```python
from build123d import *

# Parameters (mm, degrees)
BOSS_EXTRUDE1_DEPTH = 2.54
BOSS_EXTRUDE2_DEPTH = 2.54
SKETCH5_W           = 25.908
SKETCH5_H           = 34.036
BOSS_EXTRUDE3_DEPTH = 12.7
SKETCH6_R           = 1.27
BOSS_EXTRUDE4_DEPTH = 5.08
SKETCH7_W           = 5.08
SKETCH7_H           = 138.176
CUT_EXTRUDE1_DEPTH  = 2.54
CUT_EXTRUDE2_DEPTH  = 2.54


with BuildPart() as part:
    # Sketch1 → Boss-Extrude1 (new body)
    with BuildSketch(Plane(origin=(0, 0, 0), x_dir=(1, 0, 0), z_dir=(0, 1, 0))):
        Polygon((0, 0), (0, 152.4), (116.84, 152.4), (143.709327723, 0.01647018), align=None)
    extrude(amount=BOSS_EXTRUDE1_DEPTH)

    # Sketch2 → Boss-Extrude2 (add)
    with BuildSketch(Plane(origin=(0, 2.54, 0), x_dir=(1, 0, 0), z_dir=(0, 1, 0))):
        Polygon((117.220689951, 150.241), (2.159, 150.241), (2.159, 2.159), (143.331541909, 2.159), (142.435800847, 7.239), (7.239, 7.239), (7.239, 145.161), (118.116431013, 145.161), align=None)
    extrude(amount=BOSS_EXTRUDE2_DEPTH)

    # Sketch5 → Boss-Extrude3 (add)
    with BuildSketch(Plane.XZ):
        with Locations((44.90593, -61.477652)):
            Rectangle(SKETCH5_W, SKETCH5_H)
    extrude(amount=-BOSS_EXTRUDE3_DEPTH)

    # Sketch6 → Boss-Extrude4 (add)
    with BuildSketch(Plane(origin=(0, 12.7, 0), x_dir=(1, 0, 0), z_dir=(0, 1, 0))):
        with Locations((34.625191146, 75.319771658)):
            Circle(SKETCH6_R)
        with Locations((55.169983581, 75.290564093)):
            Circle(SKETCH6_R)
        with Locations((55.199191146, 49.284771658)):
            Circle(SKETCH6_R)
        with Locations((34.625191146, 49.284771658)):
            Circle(SKETCH6_R)
    extrude(amount=BOSS_EXTRUDE4_DEPTH)

    # Mirror2: part across plane


with BuildPart() as part_1:
    add(part.part)
    add(part.part.mirror(Plane(origin=(116.84, 2.54, -152.4), x_dir=(0.173648178, 0, 0.984807753), z_dir=(0.984807753, 0, -0.173648178))))

    # Sketch7 → Cut-Extrude1 (cut)
    with BuildSketch(Plane(origin=(0, 5.08, 0), x_dir=(1, 0, 0), z_dir=(0, 1, 0))):
        with Locations((4.699, 79.248)):
            Rectangle(SKETCH7_W, SKETCH7_H)
    extrude(amount=-CUT_EXTRUDE1_DEPTH, mode=Mode.SUBTRACT)

    # Sketch8 → Cut-Extrude2 (cut)
    with BuildSketch(Plane(origin=(0, 5.08, 0), x_dir=(1, 0, 0), z_dir=(0, 1, 0))):
        Polygon((86.740689951, 150.241), (86.740689951, 145.161), (118.116431013, 145.161), (140.439525591, 153.285941963), (138.702063263, 158.059580476), (117.220689951, 150.241), align=None)
    extrude(amount=-CUT_EXTRUDE2_DEPTH, mode=Mode.SUBTRACT)


solid = part_1.part
```
CAD build for the part. Positions are in the model's coordinates, mm. A direction names the side the tool comes from. Give positions to 0.01 mm unless a question says otherwise; leave off trailing zeros. Write each loop counter-clockwise with the first axis right and the second up, starting at its lowest first coordinate (ties: lowest second). Pieces come first, ordered by that corner, then holes. Notation, with made-up numbers: M 83,73.25 L 138,73.25 A12 cw 138,85.25 Z; hole C 78.5,31.5 d8. An arc over 180 degrees is marked long. Return JSON: item names as keys, results as strings. Group by question number.
(1) Band-saw the part on A-A (y = 8.5). Give the cut face in (x, z) (3 decimals), and give its area (3 significant figures).
(2) 3-axis set-ups, long thin cutter, end or side, ignore diameter. For faces 5 (the face through (210.59, 3.79, -26.64)), 6 (the face through (57.86, 8, -62)), 7 (the face through (250.312, 3.792, -120.993)), 8 (the face through (31.952, 8, -62)): which of +Z, -Z, +X, -X, +Y, -Y reach the whole face in a straight line?
(3) Band-saw the part on C-C (x = 159). Give the cut face in (y, z).
(4) Flat gauge pins, fed straight in: pin 1 Ø11 at (x, z) = (216, -93.5) entering from +Y; pin 2 Ø0.8 at (x, y) = (58.5, 4) entering from -Z; pin 3 Ø2 at (y, z) = (4.5, -149) entering from -X. Where does each tip first touch, or does it go through?
(5) Band-saw the part on B-B (z = -65). Give the cut face in (x, y).
(6) Band-saw the part on D-D (z = -29). Give the cut face in (x, y).
(7) Drill centre lines: L1, parallel to Z at x = 34.5, y = 14.75; L2, parallel to Z at x = 99.5, y = 1; L3, parallel to Y at x = 221.5, z = -83. Where is each one in solid material? Low to high. Write a range as [from, to].
(8) Mould opens along X. For faces 1 (the face through (172.505, 1.252, -172.661)), 2 (the face through (253.06, 1.252, -119.755)), 3 (the face through (221.524, 7.549, -75.634)), 4 (the face through (204, 5.08, -28)) say: pulls with the +X half, pulls with the -X half, needs draft (parallel to the pull), parting line crosses it, or undercut.
Entries:
{
 "1": {"outline": "M 31.952,-78.496 L 57.86,-78.496 L 57.86,-44.46 L 31.952,-44.46 Z; M 197.54,-103.125 L 221.885,-111.986 L 233.526,-80.003 L 209.181,-71.142 Z", "area": "1,760 mm^2"},
 "2": {"face 5": "+Z, +X, +Y", "face 6": "+Y", "face 7": "-Z, +X, +Y", "face 8": "-X, +Y"},
 "3": {"outline": "M 0,-167.74 L 2.54,-167.74 L 2.54,-165.45 L 5.08,-165.45 L 5.08,-160.04 L 2.54,-160.04 L 2.54,-13.27 L 5.08,-13.27 L 5.08,-7.86 L 2.54,-7.86 L 2.54,-5.58 L 0,-5.58 Z"},
 "4": {"pin 1": "stops at y = 12.7", "pin 2": "stops at z = -150.24", "pin 3": "stops at x = 2.16"},
 "5": {"outline": "M 0,0 L 272.99,0 L 272.99,2.54 L 270.69,2.54 L 270.69,5.08 L 265.29,5.08 L 265.29,2.54 L 57.86,2.54 L 57.86,12.7 L 31.95,12.7 L 31.95,2.54 L 0,2.54 Z"},
 "6": {"outline": "M 0,0 L 223.37,0 L 223.37,2.54 L 217.08,2.54 L 217.08,5.08 L 202.22,5.08 L 202.22,2.54 L 0,2.54 Z"},
 "7": {"L1": "z = [-76.58, -74.06], [-50.55, -48.02]", "L2": "z = [-152.4, -0.01]", "L3": "y = [0, 12.7]"},
 "8": {"face 1": "pulls with the -X half", "face 2": "pulls with the +X half", "face 3": "undercut", "face 4": "needs draft"}
}
